Input: part model. Units: mm. Frame: model coordinates. Face numbers are marked on the shaded views. A direction names the side the tool comes from. Give positions to 0.01 mm unless a question says otherwise; leave off trailing zeros. Loops run counter-clockwise (first coordinate to the right, second up) from the corner with the lowest first, then second, coordinate; pieces in that order, holes last. Notation, with made-up numbers: M 0.25,37 L 37.25,37 A27 ccw 37.25,54 Z; hole C -9.5,81 d8. An arc over 180 degrees is marked long. One line per item, written item: value. Start each with the question number.
(1) Section A-A on x = -44.45. Output: boundary loops of the cut face in (y, z).
(2) Section B-B on y = 0. Output: boundary loops of the cut face in (x, z), plus the area to 3 significant figures.
(3) Section C-C on z = 23.5. Output: boundary loops of the cut face in (x, y), plus the area to 3 significant figures.
(4) Ray query, line 1 along X through (y, z) = (0, 3); line 2 along Y through (x, z) = (44.45, 10); line 3 along X through (y, z) = (0, 5.5). Return the intervals inside material, ascending. Write a range as from..to.
(5) Pull-direction query (X, two-part tool) for the marked faces 1, 2 and 3; classes: released by +X, released by -X, zero draft, split by the parting line, or undercut.
(6) Pin query (flat end, axial travel): P1, Ø16.5, axis at x = 51.5, y = -7.5, coming from the +Z side; P2, Ø1, axis at y = 11, z = 22.5, coming from the -X side; P3, Ø3, axis at y = 9, z = 29, coming from the -X side; P4, Ø6, axis at x = 5.5, y = -7.5, coming from the -Z side. Return the tip coordinate at first contact, or that it passes through.
(7) Section D-D on z = 9. Output: boundary loops of the cut face in (x, y).
(8) Access query for the marked faces 4, 5 and 6. Directions: +Z, -Z, +X, -X, +Y, -Y. A direction counts if a zero-diameter tool reaches every point of the face in a straight line with its end or side. Return the directions, or none.
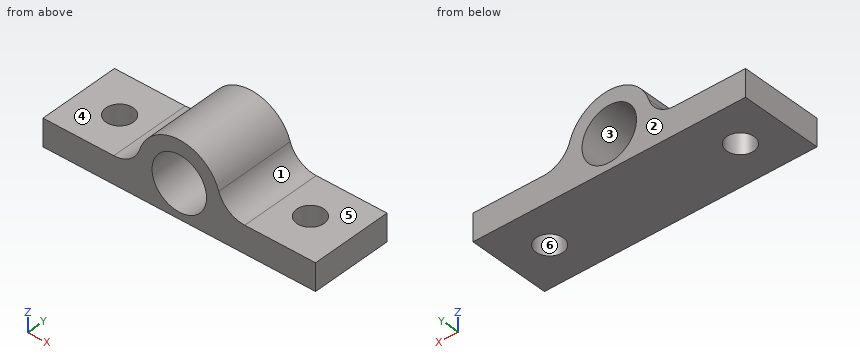
```python
from build123d import *

# Parameters (mm, degrees)
F0_R     = 12.7
F1_DEPTH = 19.05
F2_R     = 12.7
F3_R     = 6.35
F5_DEPTH = 12.7


# Not quite as in the source:
# - the program builds the solid bodies; features that only make, move or delete a surface that nothing else refers to are left out


with BuildPart() as f1:
    # F0 (on Front) → F1 (new body, symmetric)
    with BuildSketch(Plane.XZ):
        with BuildLine():
            Line((-63.5, 12.7), (-63.5, 0))
            Line((-63.5, 0), (63.5, 0))
            Line((63.5, 0), (63.5, 12.7))
            Line((63.5, 12.7), (19.05, 12.7))
            ThreePointArc((19.05, 12.7), (0, 35.1124285501), (-19.05, 12.7))
            Line((-19.05, 12.7), (-63.5, 12.7))
        make_face()
        with Locations((0, 15.8102040816)):
            Circle(F0_R, mode=Mode.SUBTRACT)
    extrude(amount=F1_DEPTH, both=True)

    # F2
    f2_edges = [f1.edges().sort_by_distance(p)[0] for p in [
        (-19.05, 0, 12.7),
        (19.05, 0, 12.7),
    ]]
    fillet(f2_edges, radius=F2_R)

    # F3 (on face) → F5 (cut, through all)
    with BuildSketch(Plane(origin=(0, 0, 0), x_dir=(1, 0, 0), z_dir=(0, 0, -1))):
        with Locations((-44.45, 0)):
            Circle(F3_R)
        with Locations((44.45, 0)):
            Circle(F3_R)
    extrude(amount=-F5_DEPTH, mode=Mode.SUBTRACT)


solid = f1.part
```
Output values:
1. outline: M -19.05,0 L -6.35,0 L -6.35,12.7 L -19.05,12.7 Z; M 6.35,0 L 19.05,0 L 19.05,12.7 L 6.35,12.7 Z
2. outline: M -63.5,0 L -50.8,0 L -50.8,12.7 L -63.5,12.7 Z; M -38.1,0 L 38.1,0 L 38.1,12.7 L 30.53,12.7 A12.7 cw 18.42,21.59 A19.3 ccw -18.42,21.59 A12.7 cw -30.53,12.7 L -38.1,12.7 Z; M 50.8,0 L 63.5,0 L 63.5,12.7 L 50.8,12.7 Z; hole C 0,15.81 d25.4
2. area: 1,530 mm²
3. outline: M -17.7,-19.05 L -10.11,-19.05 L -10.11,19.05 L -17.7,19.05 Z; M 10.11,-19.05 L 17.7,-19.05 L 17.7,19.05 L 10.11,19.05 Z
3. area: 579 mm²
4. line 1: x = -63.5..-50.8, -38.1..38.1, 50.8..63.5
4. line 2: y = -19.05..-6.35, 6.35..19.05
4. line 3: x = -63.5..-50.8, -38.1..-7.42, 7.42..38.1, 50.8..63.5
5. face 1: released by +X
5. face 2: zero draft
5. face 3: undercut
6. P1: stops at z = 12.7
6. P2: stops at x = -18.28
6. P3: stops at x = -15.36
6. P4: stops at z = 0
7. outline: M -63.5,-19.05 L -10.72,-19.05 L -10.72,19.05 L -63.5,19.05 Z; M 10.72,-19.05 L 63.5,-19.05 L 63.5,19.05 L 10.72,19.05 Z; hole C -44.45,0 d12.7; hole C 44.45,0 d12.7
8. face 4: +Z, -X, +Y, -Y
8. face 5: +Z, +X, +Y, -Y
8. face 6: +Z, -Z
